Verification items for the finished model (mm, model axes). Face numbers are marked on the shaded views. A direction names the side the tool comes from. Round coordinates to 2 decimals unless told otherwise and drop trailing zeros. Write each loop counter-clockwise with the first axis right and the second up, starting at its lowest first coordinate (ties: lowest second). Pieces come first, ordered by that corner, then holes.
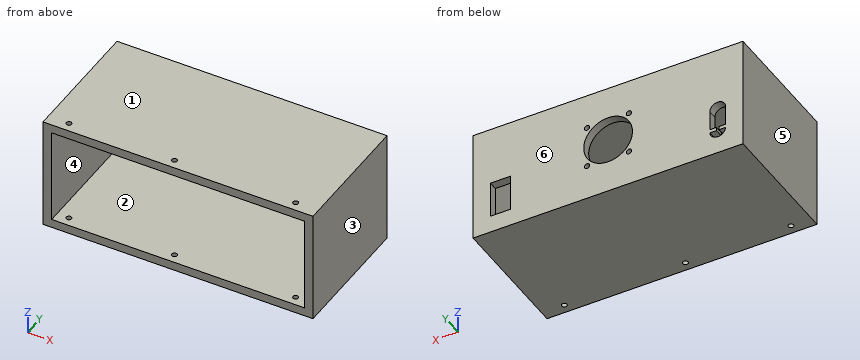
from build123d import *

# Parameters (mm, degrees)
SKETCH1_W           = 155
SKETCH1_H           = 65
BOSS_EXTRUDE2_DEPTH = 75
SKETCH2_W           = 145
SKETCH2_H           = 55
CUT_EXTRUDE1_DEPTH  = 70
SKETCH3_R           = 14
SKETCH3_R_2         = 1.5
SKETCH3_W           = 11.5
SKETCH3_H           = 21
CUT_EXTRUDE2_DEPTH  = 70
SKETCH5_R           = 1.5
CUT_EXTRUDE3_DEPTH  = 73
SKETCH6_W           = 3.75
SKETCH6_H           = 2
BOSS_EXTRUDE3_DEPTH = 5


with BuildPart() as part:
    # Sketch1 → Boss-Extrude2 (new body)
    with BuildSketch(Plane(origin=(0, 0, 0), x_dir=(1, 0, 0), z_dir=(0, 1, 0))):
        with Locations((-63.409090909, -25.909090909)):
            Rectangle(SKETCH1_W, SKETCH1_H)
    extrude(amount=BOSS_EXTRUDE2_DEPTH)

    # Sketch2 → Cut-Extrude1 (cut)
    with BuildSketch(Plane.XZ):
        with Locations((-63.409090909, 25.909090909)):
            Rectangle(SKETCH2_W, SKETCH2_H)
    extrude(amount=-CUT_EXTRUDE1_DEPTH, mode=Mode.SUBTRACT)

    # Sketch3 → Cut-Extrude2 (cut)
    with BuildSketch(Plane(origin=(0, 75, 0), x_dir=(1, 0, 0), z_dir=(0, 1, 0))):
        with Locations(Location((-63.480160731, -25.837348529, 0), (0, 0, 270))):
            Circle(SKETCH3_R)
        with Locations(Location((-75.444232667, -13.760056502, 0), (0, 0, 270))):
            Circle(SKETCH3_R_2)
        with Locations(Location((-51.373949151, -13.760056502, 0), (0, 0, 90))):
            Circle(SKETCH3_R_2)
        with Locations(Location((-51.373949151, -38.058125316, 0), (0, 0, 270))):
            Circle(SKETCH3_R_2)
        with Locations(Location((-75.444232667, -38.058125316, 0), (0, 0, 90))):
            Circle(SKETCH3_R_2)
        with BuildLine():
            Line((-121.909090909, -7.909090909), (-121.909090909, -20.909090909))
            ThreePointArc((-121.909090909, -20.909090909), (-126.409090909, -25.409090909), (-130.909090909, -20.909090909))
            Line((-130.909090909, -20.909090909), (-130.909090909, -7.909090909))
            ThreePointArc((-130.909090909, -7.909090909), (-126.409090909, -3.409090909), (-121.909090909, -7.909090909))
        make_face()
        with Locations((-1.659090909, -13.909090909)):
            Rectangle(SKETCH3_W, SKETCH3_H)
    extrude(amount=-CUT_EXTRUDE2_DEPTH, mode=Mode.SUBTRACT)

    # Sketch5 → Cut-Extrude3 (cut)
    with BuildSketch(Plane.XY.offset(58.409090909)):
        with Locations((-68.4120524, 5.312033368)):
            Circle(SKETCH5_R)
        with Locations((1.156357058, 5.323906477)):
            Circle(SKETCH5_R)
        with Locations((-129.008167682, 5.312033368)):
            Circle(SKETCH5_R)
    extrude(amount=-CUT_EXTRUDE3_DEPTH, mode=Mode.SUBTRACT)

    # Sketch6 → Boss-Extrude3 (add)
    with BuildSketch(Plane(origin=(0, 75, 0), x_dir=(1, 0, 0), z_dir=(0, 1, 0))):
        with Locations((-129.034090909, -8.609090909)):
            Rectangle(SKETCH6_W, SKETCH6_H)
        with Locations((-123.784090909, -8.609090909)):
            Rectangle(SKETCH6_W, SKETCH6_H)
    extrude(amount=-BOSS_EXTRUDE3_DEPTH)


solid = part.part
Q1. Material ranges on line 1 along X through (y, z) = (56, 9); line 2 along Z through (x, y) = (-129, 57); line 3 along Y through (x, z) = (-21.5, 20.5), recorded low to high.
Recorded:
line 1: x = -140.91 to -135.91, 9.09 to 14.09
line 2: z = -6.59 to -1.59, 53.41 to 58.41
line 3: y = 70 to 75
Q2. Sectioned sample at C-C (z = 44). Enter the section's corners in (x, y), plus the area to 4 significant figures.
Recorded:
outline: (-140.91, 0) - (-135.91, 0) - (-135.91, 70) - (9.09, 70) - (9.09, 0) - (14.09, 0) - (14.09, 75) - (-140.91, 75) - close
area: 1,475 mm2
Q3. Sectioned sample at A-A (y = 52.5). Enter the section's corners in (x, z).
Recorded:
outline: (-140.91, -6.59) - (14.09, -6.59) - (14.09, 58.41) - (-140.91, 58.41) - close; hole (-135.91, -1.59) - (9.09, -1.59) - (9.09, 53.41) - (-135.91, 53.41) - close
Q4. Sectioned sample at B-B (x = -108.5). Enter the section's corners in (y, z).
Recorded:
outline: (0, -6.59) - (75, -6.59) - (75, 58.41) - (0, 58.41) - (0, 53.41) - (70, 53.41) - (70, -1.59) - (0, -1.59) - close
Q5. Tool access check on the marked faces 1 and 2. Record the directions out of +Z, -Z, +X, -X, +Y, -Y that give a thin tool (end or side, any length) a straight path to the whole face; none if there is none.
Recorded:
face 1: +Z, +X, -X, +Y, -Y
face 2: -Y
Q6. Release check for a two-part mould opening along X. For the marked faces 3, 4, 5 and 6 record: released by +X, released by -X, zero draft, split by the parting line, or undercut.
Recorded:
face 3: released by +X
face 4: undercut
face 5: released by -X
face 6: zero draft
Q7. Depth check by flat-ended pin: P1, Ø1, axis at x = -20, z = 36.5, coming from the -Y side. Enter the tip coordinate at first touch or a pass-through.
Recorded:
P1: stops at y = 70
